```python
from build123d import *

# Parameters (mm, degrees)
SKETCH1_R           = 2.55
BOSS_EXTRUDE1_DEPTH = 6.35


with BuildPart() as part:
    # Sketch1 → Boss-Extrude1 (new body)
    with BuildSketch(Plane(origin=(0, 0, 0), x_dir=(1, 0, 0), z_dir=(0, 1, 0))):
        with BuildLine():
            Line((0, -42.5), (-35, -42.5))
            Line((-35, -42.5), (-35, -30.733037331))
            ThreePointArc((-35, -30.733037331), (-21.855245126, 0), (-35, 30.733037331))
            Line((-35, 30.733037331), (-35, 42.5))
            Line((-35, 42.5), (0, 42.5))
            Line((0, 42.5), (33.5, 42.5))
            Line((33.5, 42.5), (33.5, 32.5))
            Line((33.5, 32.5), (33.5, 30.733037331))
            ThreePointArc((33.5, 30.733037331), (20.355245126, 0), (33.5, -30.733037331))
            Line((33.5, -30.733037331), (33.5, -32.5))
            Line((33.5, -32.5), (33.5, -42.5))
            Line((33.5, -42.5), (0, -42.5))
        make_face()
        with Locations(Location((-30.75, -32.5, 0), (0, 0, 270))):
            Circle(SKETCH1_R, mode=Mode.SUBTRACT)
        with Locations(Location((-30.75, 32.5, 0), (0, 0, 270))):
            Circle(SKETCH1_R, mode=Mode.SUBTRACT)
        with Locations(Location((-10.75, 32.5, 0), (0, 0, 270))):
            Circle(SKETCH1_R, mode=Mode.SUBTRACT)
        with Locations(Location((-10.75, -32.5, 0), (0, 0, 270))):
            Circle(SKETCH1_R, mode=Mode.SUBTRACT)
        with BuildLine():
            Line((29.25, -35), (19.25, -35))
            ThreePointArc((19.25, -35), (16.75, -32.5), (19.25, -30))
            Line((19.25, -30), (29.25, -30))
            ThreePointArc((29.25, -30), (31.75, -32.5), (29.25, -35))
        make_face(mode=Mode.SUBTRACT)
        with BuildLine():
            Line((9.25, -35), (-0.75, -35))
            ThreePointArc((-0.75, -35), (-3.25, -32.5), (-0.75, -30))
            Line((-0.75, -30), (9.25, -30))
            ThreePointArc((9.25, -30), (11.75, -32.5), (9.25, -35))
        make_face(mode=Mode.SUBTRACT)
        with BuildLine():
            Line((29.25, 30), (19.25, 30))
            ThreePointArc((19.25, 30), (16.75, 32.5), (19.25, 35))
            Line((19.25, 35), (29.25, 35))
            ThreePointArc((29.25, 35), (31.75, 32.5), (29.25, 30))
        make_face(mode=Mode.SUBTRACT)
        with BuildLine():
            Line((9.25, 30), (-0.75, 30))
            ThreePointArc((-0.75, 30), (-3.25, 32.5), (-0.75, 35))
            Line((-0.75, 35), (9.25, 35))
            ThreePointArc((9.25, 35), (11.75, 32.5), (9.25, 30))
        make_face(mode=Mode.SUBTRACT)
    extrude(amount=-BOSS_EXTRUDE1_DEPTH)


solid = part.part
```
Check sheet for the modelled part. Datum: model origin and axes. Units: mm. A direction names the side the tool comes from. Give positions to 0.01 mm unless a question says otherwise; leave off trailing zeros. Write each loop counter-clockwise with the first axis right and the second up, starting at its lowest first coordinate (ties: lowest second). Pieces come first, ordered by that corner, then holes.
Item 1: Scan lines: L1, parallel to X at y = -4, z = -32.5; L2, parallel to Z at x = 2, y = -4; L3, parallel to X at y = -3.5, z = 30.5. Record each from-to range of solid material in increasing order.
Item 2: Gauge pin test, flat ends, axial feed: pin 1 (1 mm diameter, centred on y = -3, z = 8, fed in from +X); pin 2 (3 mm diameter, centred on x = -30.75, z = 32.5, fed in from +Y); pin 3 (2 mm diameter, centred on y = -5.5, z = 25, fed in from +X). Record the tip position at first contact, or that the pin passes through.
Item 3: Cross-section at B-B (z = -32.5). Enter the section's corners in (x, y).
Item 4: Draft check along Z on faces 1 (the face through (33.5, -3, -37)), 2 (the face through (-1, -3, -42.5)), 3 (the face through (24, -3, -35)). Enter one of: released by +Z, released by -Z, zero draft, split by the parting line, or undercut.
Item 5: Cross-section at C-C (y = -4.25). Count the separate pieces of the cut face and the enclosed holes in it, and give its area (3 significant figures).
Item 6: Access from +Z, -Z, +X, -X, +Y, -Y to the whole of each face (thin tool, end or side, straight path). Record for faces 4 (the face through (16.75, -3.13, -32.45)), 5 (the face through (0, -6.35, -1)).
Item 7: Cross-section at D-D (x = 7). Enter the section's corners in (y, z).
Item 8: Cross-section at A-A (x = -10.75). Enter the section's corners in (y, z), and give its area (3 significant figures).
Report:
1. L1: x = -35 to -33.3, -28.2 to -13.3, -8.2 to -3.25, 11.75 to 16.75, 31.75 to 33.5
1. L2: z = -42.5 to -35, -30 to 30, 35 to 42.5
1. L3: x = -34.76 to -32.33, -29.17 to -12.33, -9.17 to -2.25, 10.75 to 17.75, 30.75 to 33.26
2. pin 1: stops at x = 21.21
2. pin 2: passes through
2. pin 3: stops at x = 29.24
3. outline: (-35, -6.35) - (-33.3, -6.35) - (-33.3, 0) - (-35, 0) - close; (-28.2, -6.35) - (-13.3, -6.35) - (-13.3, 0) - (-28.2, 0) - close; (-8.2, -6.35) - (-3.25, -6.35) - (-3.25, 0) - (-8.2, 0) - close; (11.75, -6.35) - (16.75, -6.35) - (16.75, 0) - (11.75, 0) - close; (31.75, -6.35) - (33.5, -6.35) - (33.5, 0) - (31.75, 0) - close
4. face 1: zero draft
4. face 2: released by -Z
4. face 3: undercut
5. separate pieces: 1
5. enclosed holes: 8
5. area: 4,350 mm2
6. face 4: +Y, -Y
6. face 5: +Z, -Z, +X, -X, -Y
7. outline: (-6.35, -42.5) - (0, -42.5) - (0, -35) - (-6.35, -35) - close; (-6.35, -30) - (0, -30) - (0, 30) - (-6.35, 30) - close; (-6.35, 35) - (0, 35) - (0, 42.5) - (-6.35, 42.5) - close
8. outline: (-6.35, -42.5) - (0, -42.5) - (0, -35.05) - (-6.35, -35.05) - close; (-6.35, -29.95) - (0, -29.95) - (0, 29.95) - (-6.35, 29.95) - close; (-6.35, 35.05) - (0, 35.05) - (0, 42.5) - (-6.35, 42.5) - close
8. area: 475 mm2
